Could you check a few things on this model? Use its own coordinates, in mm. Face numbers are marked on the shaded views. Round coordinates to 2 decimals unless told otherwise and drop trailing zeros. Write each loop counter-clockwise with the first axis right and the second up, starting at its lowest first coordinate (ties: lowest second). Pieces come first, ordered by that corner, then holes. Notation, with made-up numbers: (48.25, -14.5) -> (86.25, -14.5) arc R24 cw to (86.25, -0.5) -> close; hole circle Ø3 at (35.5, 44.5). An arc over 180 degrees is marked (long way). One line per question, with ' | ' between items. Start each with the question number.
1. Thinking about a two-plate mould opening in Y: for the marked faces 1 and 2, which applies, released by +Y, released by -Y, zero draft, split by the parting line, or undercut?
2. Imagine slicing it at D-D, the plane z = 27.5. List the corners of the cut face in (x, y) for me, and give its area (3 significant figures).
3. Imagine slicing it at A-A, the plane x = 0. List the corners of the cut face in (y, z) for me, and give its area (3 significant figures).
4. For pin 1 Ø8 at (y, z) = (-26.5, 5) entering from +X; pin 2 Ø10 at (x, y) = (-77.5, -64) entering from -Z; pin 3 Ø4 at (y, z) = (73, 18.5) entering from +X; pin 4 Ø1.5 at (y, z) = (-29.5, 6) entering from -X, each with a flat end and sliding along its axis, tell me the tip position at first contact or that it passes through.
5. If I drill on line 1 along X through (y, z) = (2.5, 3.5); line 2 along Y through (x, z) = (0, 24.75); line 3 along X through (y, z) = (66, 10), over which ranges is the centre line in solid material (lowest first)? Write a range as [from, to].
6. Imagine slicing it at C-C, the plane z = 7. List the corners of the cut face in (x, y) for me.
from build123d import *

# Parameters (mm, degrees)
F0_R     = 99.4
F0_R_2   = 97
F1_DEPTH = 20
F2_R     = 99.4
F2_R_2   = 95.4
F3_DEPTH = 12
F4_SIZE  = 0.4
F5_SIZE  = 0.5


with BuildPart() as f1:
    # F0 (on Top) → F1 (new body)
    with BuildSketch(Plane.XY):
        Circle(F0_R)
        Circle(F0_R_2, mode=Mode.SUBTRACT)
    extrude(amount=F1_DEPTH)

    # F2 (on face) → F3 (join)
    with BuildSketch(Plane.XY.offset(20)):
        Circle(F2_R)
        Circle(F2_R_2, mode=Mode.SUBTRACT)
    extrude(amount=F3_DEPTH)

    # F4
    f4_edges = [f1.edges().sort_by_distance(p)[0] for p in [
        (-99.4, 0, 32),
        (-95.4, 0, 32),
    ]]
    chamfer(f4_edges, length=F4_SIZE)

    # F5
    f5_edges = [f1.edges().sort_by_distance(p)[0] for p in [
        (-99.4, 0, 0),
    ]]
    chamfer(f5_edges, length=F5_SIZE)


solid = f1.part
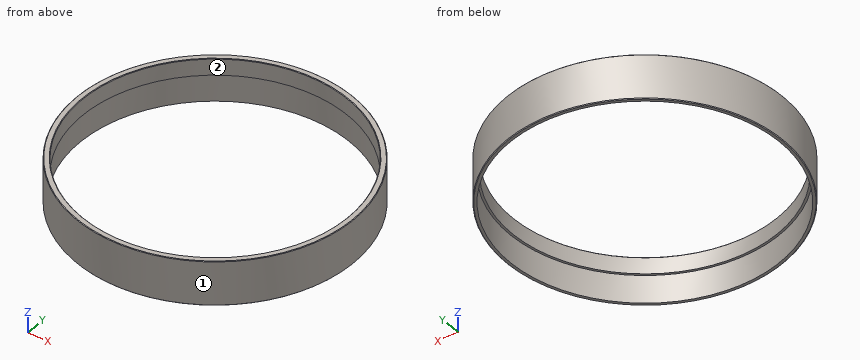
Geometry results:
1) face 1: split by the parting line | face 2: undercut
2) outline: circle Ø198.8 at (0, 0); hole circle Ø190.8 at (0, 0) | area: 2,450 mm2
3) outline: (-99.4, 0.5) -> (-98.9, 0) -> (-97, 0) -> (-97, 20) -> (-95.4, 20) -> (-95.4, 31.6) -> (-95.8, 32) -> (-99, 32) -> (-99.4, 31.6) -> close; (95.4, 20) -> (97, 20) -> (97, 0) -> (98.9, 0) -> (99.4, 0.5) -> (99.4, 31.6) -> (99, 32) -> (95.8, 32) -> (95.4, 31.6) -> close | area: 191 mm2
4) pin 1: stops at x = 96.82 | pin 2: stops at z = 0 | pin 3: stops at x = 69.57 | pin 4: stops at x = -95.15
5) line 1: x = [-99.37, -96.97], [96.97, 99.37] | line 2: y = [-99.4, -95.4], [95.4, 99.4] | line 3: x = [-74.33, -71.08], [71.08, 74.33]
6) outline: circle Ø198.8 at (0, 0); hole circle Ø194 at (0, 0)
